Here's the drawing with two shaded views (mm, measured from the low corner). I have some questions. Coordinates: 2 decimals unless noted, no trailing zeros. Loops run counter-clockwise (first coordinate to the right, second up) from the corner with the lowest first, then second, coordinate; pieces in that order, holes last. Notation, with made-up numbers: (1.25, -23) -> (37.25, -23) arc R19 cw to (37.25, -13) -> close; hole circle Ø7 at (83, 14). An arc over 180 degrees is marked (long way). Answer as a JSON object with one key per item and string values. Group by question number.
1) I'm going to push a flat-ended pin straight in: pin 1 (2.5 mm diameter, centred on x = 70.29, z = 52, fed in from +Y). Where does the tip first touch, or does it pass through?
2) I want a section at B-B (x = 12). Write out the boundary of the cut face in (y, z).
3) I want a section at A-A (y = 0.2). Write out the boundary of the cut face in (x, z) (1 decimal), then the cut area to 3 significant figures.
4) I need wall thicknesses on probe 1 along X at (y, z) = (0.75, 18.5) (1 decimal); probe 2 along X at (y, z) = (0.1, 22.5) (1 decimal); probe 3 along Z at (x, y) = (24, 0.1) (1 decimal). Which ranges of each line are inside material? Lowest first, please. Write a range as [from, to].
5) I want a section at C-C (z = 26). Write out the boundary of the cut face in (x, y).
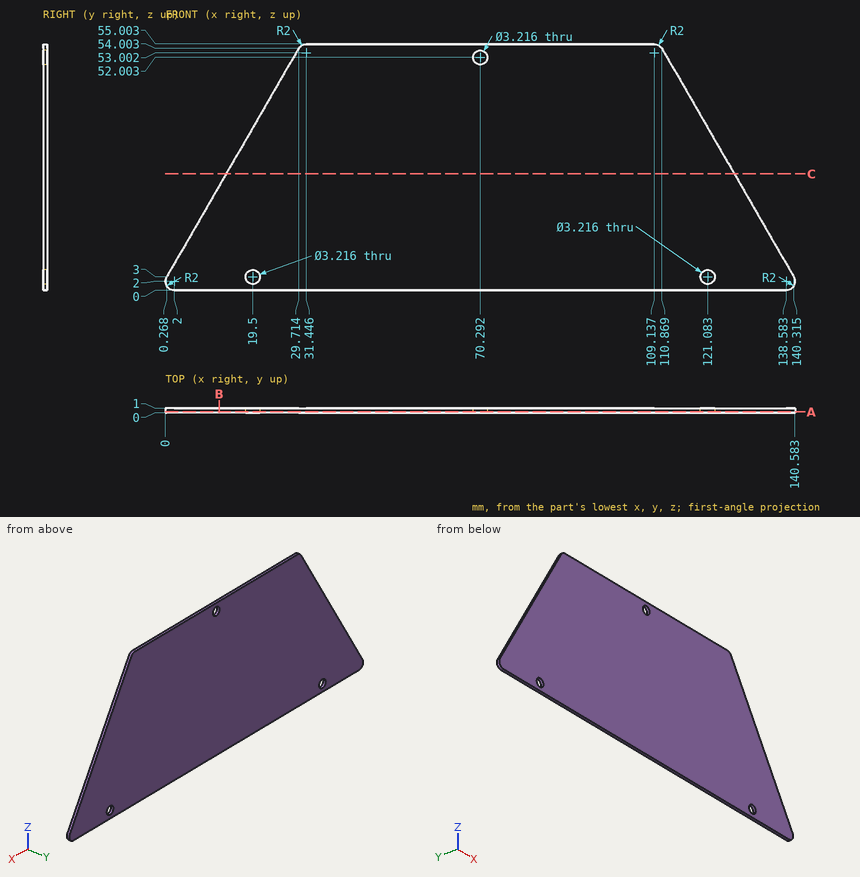
Determined:
{
 "1": {"pin 1": "through"},
 "2": {"outline": "(0, 0) -> (1, 0) -> (1, 23.32) -> (0, 23.32) -> close"},
 "3": {"outline": "(0.3, 3) arc R2 ccw to (2, 0) -> (138.6, 0) arc R2 ccw to (140.3, 3) -> (110.9, 54) arc R2 ccw to (109.1, 55) -> (31.4, 55) arc R2 ccw to (29.7, 54) -> close; hole circle Ø3.2 at (19.5, 3); hole circle Ø3.2 at (70.3, 52); hole circle Ø3.2 at (121.1, 3)", "area": "6,120 mm^2"},
 "4": {"probe 1": "[9.2, 131.4]", "probe 2": "[11.5, 129.1]", "probe 3": "[0, 44.1]"},
 "5": {"outline": "(13.55, 0) -> (127.04, 0) -> (127.04, 1) -> (13.55, 1) -> close"}
}
